Could you check a few things on this model? Use its own coordinates, in mm. A direction names the side the tool comes from. Give positions to 0.01 mm unless a question says otherwise; leave off trailing zeros. Loops run counter-clockwise (first coordinate to the right, second up) from the corner with the lowest first, then second, coordinate; pieces in that order, holes last. Notation, with made-up numbers: (69, -10) - (112, -10) arc R8 ccw to (112, -2) - close; hole circle Ø1 at (-11.5, 2.5). An arc over 180 degrees is marked (long way). Use CSV: the item, a comma, the result in double quotes.
from build123d import *

# Parameters (mm, degrees)
ESBO_O1_R                     = 1.6
RESSALTO_EXTRUS_O1_DEPTH      = 5
RESSALTO_EXTRUS_O1_2_DEPTH    = 5
RESSALTO_EXTRUS_O2_DEPTH      = 8
RESSALTO_EXTRUS_O2_DEPTH_BACK = 5
ESBO_O3_R                     = 1.65
CORTE_EXTRUS_O1_DEPTH         = 23
CORTE_EXTRUS_O1_DEPTH_BACK    = 11


with BuildPart() as part:
    # Esbo_o1 → Ressalto-extrus_o1 (new body)
    with BuildSketch(Plane.XY):
        with BuildLine():
            ThreePointArc((-4, -0.9), (-0.051399019, -4.099677809), (3.97617907, -1))
            Line((3.97617907, -1), (8, -1))
            Line((8, -1), (8, -16))
            Line((8, -16), (-4, -16))
            Line((-4, -16), (-4, -0.9))
        make_face()
        with Locations((2, -11)):
            Circle(ESBO_O1_R, mode=Mode.SUBTRACT)
    extrude(amount=RESSALTO_EXTRUS_O1_DEPTH)



with BuildPart() as body_2:
    # Esbo_o1 → Ressalto-extrus_o1 2 (new body)
    with BuildSketch(Plane.XY):
        with BuildLine():
            ThreePointArc((3.97617907, 1), (-0.051399019, 4.099677809), (-4, 0.9))
            Line((-4, 0.9), (-4, 16))
            Line((-4, 16), (8, 16))
            Line((8, 16), (8, 1))
            Line((8, 1), (3.97617907, 1))
        make_face()
        with Locations((2, 11)):
            Circle(ESBO_O1_R, mode=Mode.SUBTRACT)
    extrude(amount=RESSALTO_EXTRUS_O1_2_DEPTH)


with BuildPart() as part_1:
    add(part.part)

    add(body_2.part)  # Ressalto-extrus_o2 merges body 2
    # Esbo_o2 → Ressalto-extrus_o2 (add, two sides)
    with BuildSketch(Plane.XY.offset(5)) as ressalto_extrus_o2_sk:
        with BuildLine():
            Line((12, 6), (12, 1))
            Line((12, 1), (3.97617907, 1))
            ThreePointArc((3.97617907, 1), (-4.1, 0), (3.97617907, -1))
            Line((3.97617907, -1), (12, -1))
            Line((12, -1), (12, -6))
            Line((12, -6), (0, -6))
            ThreePointArc((0, -6), (-6, 0), (0, 6))
            Line((0, 6), (12, 6))
        make_face()
    extrude(amount=RESSALTO_EXTRUS_O2_DEPTH)
    extrude(ressalto_extrus_o2_sk.sketch, amount=-RESSALTO_EXTRUS_O2_DEPTH_BACK)

    # Esbo_o3 → Corte-extrus_o1 (cut, two sides)
    with BuildSketch(Plane.XZ.offset(-6)) as corte_extrus_o1_sk:
        with Locations((8.35, 9)):
            Circle(ESBO_O3_R)
    extrude(amount=CORTE_EXTRUS_O1_DEPTH, mode=Mode.SUBTRACT)
    extrude(corte_extrus_o1_sk.sketch, amount=-CORTE_EXTRUS_O1_DEPTH_BACK, mode=Mode.SUBTRACT)


solid = part_1.part
1) I need wall thicknesses on line 1 along Z through (x, y) = (8.35, 4.1); line 2 along Y through (x, z) = (7.5, 3.75); line 3 along Y through (x, z) = (0, 3.25). Which ranges of each line are inside material? Lowest first, please.
Answer below:
line 1,"z = 0 to 7.35, 10.65 to 13"
line 2,"y = -16 to -1, 1 to 16"
line 3,"y = -16 to -4.1, 4.1 to 16"
2) Suppose I cut it at D-D (z = 4.5). Please give me the cut outline in (x, y), plus the area to 3 significant figures.
Answer below:
outline,"(-4, -16) - (8, -16) - (8, -6) - (12, -6) - (12, -1) - (3.98, -1) arc R4.1 cw (long way) to (3.98, 1) - (12, 1) - (12, 6) - (8, 6) - (8, 16) - (-4, 16) - (-4, 4.47) arc R6 ccw to (-4, -4.47) - close; hole circle Ø3.2 at (2, -11); hole circle Ø3.2 at (2, 11)"
area,"360 mm2"
3) I'm going to push flat-ended pins straight in: P1, Ø4, axis at x = 8.35, z = 9, coming from the +Y side; P2, Ø5.5, axis at y = -9, z = 2, coming from the +X side; P3, Ø8, axis at x = 0.5, y = -6, coming from the -Z side; P4, Ø4, axis at x = 8.5, y = -9.5, coming from the +Z side. Where does each tip first touch, or does it pass through?
Answer below:
P1,"stops at y = 6"
P2,"stops at x = 8"
P3,"stops at z = 0"
P4,"stops at z = 5"
4) Suppose I cut it at A-A (x = 5.25). Please give me the cut outline in (y, z), plus the area to 3 significant figures.
Answer below:
outline,"(-16, 0) - (-1, 0) - (-1, 13) - (-6, 13) - (-6, 5) - (-16, 5) - close; (1, 0) - (16, 0) - (16, 5) - (6, 5) - (6, 13) - (1, 13) - close"
area,"230 mm2"
5) Suppose I cut it at C-C (y = -2.5). Please give me the cut outline in (x, z).
Answer below:
outline,"(-5.45, 0) - (-3.25, 0) - (-3.25, 13) - (-5.45, 13) - close; (3.25, 0) - (12, 0) - (12, 13) - (3.25, 13) - close; hole circle Ø3.3 at (8.35, 9)"
6) Suppose I cut it at B-B (z = 9). Please give me the cut outline in (x, y), plus the area to 3 significant figures.
Answer below:
outline,"(0, -6) - (6.7, -6) - (6.7, -1) - (3.98, -1) arc R4.1 cw (long way) to (3.98, 1) - (6.7, 1) - (6.7, 6) - (0, 6) arc R6 ccw to start; (10, -6) - (12, -6) - (12, -1) - (10, -1) - close; (10, 1) - (12, 1) - (12, 6) - (10, 6) - close"
area,"98.9 mm2"
7) Which directions (+Z, -Z, +X, -X, +Y, -Y) give clear straight access to the entire face, cutting with the end or side of a thin tool? Please do faces 1 (the flat face through (8, -1, 6)), 2 (the flat face through (-4, 10, 2)), 3 (the flat face through (-4, -10, 2)).
Answer below:
face 1,"+Z, -Z, +X"
face 2,"+Z, -Z, -X, +Y"
face 3,"+Z, -Z, -X, -Y"
8) We'd pull the mould along Y, two halves only. Please class faces 4 (the cylindrical face through (0.82, 12.08, 2.46)), 5 (the flat face through (8, 11, 2)), 6 (the cylindrical face through (-6, 0, 8)): +Y half, -Y half, draft (parallel to the pull), parting line (faces both ways), or undercut.
Answer below:
face 4,"undercut"
face 5,"draft"
face 6,"parting line"
